Part model, mm, in its own coordinate system. A direction names the side the tool comes from. Round coordinates to 2 decimals unless told otherwise and drop trailing zeros. Order: outer loops, then holes, each group sorted by start corner. A loop starts at its lowest first (then second) coordinate and runs counter-clockwise, first axis right, second up. Notation, with made-up numbers: (2, 2.5) - (42, 2.5) arc R13 ccw to (42, 23.5) - close; hole circle Ø5 at (86, -39.75). An arc over 180 degrees is marked (long way). Answer as a JSON object with one key per item and string values.
```python
from build123d import *

# Parameters (mm, degrees)
FILLET1_R      = 0.1
FILLET2_R      = 0.12
CHAMFER1_SIZE  = 0.2
EXTRUDE1_DEPTH = 1.1


with BuildPart() as part:
    # Sketch1 → Revolve1 (revolve)
    with BuildSketch(Plane.XY, mode=Mode.PRIVATE) as revolve1_sk:
        Polygon((2.5, 1.25), (2.5, 0), (4.279914881, 0), (27.5, 0), (27.5, 1.25), align=None)
        Polygon((0, 2.25), (0, 0), (2.5, 0), (2.5, 1.25), (2.5, 2.25), align=None)
    revolve(revolve1_sk.sketch.rotate(Axis((0, 0, 0), (1, 0, 0)), 90), axis=Axis((0, 0, 0), (1, 0, 0)))

    # Fillet1
    fillet1_edges = [part.edges().sort_by_distance(p)[0] for p in [
        (2.5, 0, -1.25),
    ]]
    fillet(fillet1_edges, radius=FILLET1_R)

    # Fillet2
    fillet2_edges = [part.edges().sort_by_distance(p)[0] for p in [
        (0, 0, -2.25),
    ]]
    fillet(fillet2_edges, radius=FILLET2_R)

    # Chamfer1
    chamfer1_edges = [part.edges().sort_by_distance(p)[0] for p in [
        (27.5, 0, -1.25),
    ]]
    chamfer(chamfer1_edges, length=CHAMFER1_SIZE)

    # Sketch2 → Extrude1 (cut)
    with BuildSketch(Plane.ZY):
        Polygon((0, 1.154700538), (-1, 0.577350269), (-1, -0.577350269), (0, -1.154700538), (1, -0.577350269), (1, 0.577350269), align=None)
    extrude(amount=-EXTRUDE1_DEPTH, mode=Mode.SUBTRACT)


solid = part.part
```
Item 1: Tool access for faces 1 (the flat face through (27.5, 0, 0)), 2 (the flat face through (0.5, 0, -1)), 3 (the cylindrical face through (14.78, -0.05, -1.25)): list every direction of +Z, -Z, +X, -X, +Y, -Y with a clear straight run to the whole face (end or side of a thin tool).
Taken from the geometry:
{"face 1": "+Z, -Z, +X, +Y, -Y", "face 2": "-X", "face 3": "+X"}
Item 2: Cut at A-A (y = 0). Write the cut outline in (x, z), plus the area to 3 significant figures.
Taken from the geometry:
{"outline": "(0, -2.13) arc R0.12 ccw to (0.12, -2.25) - (2.5, -2.25) - (2.5, -1.35) arc R0.1 cw to (2.6, -1.25) - (27.3, -1.25) - (27.5, -1.05) - (27.5, 1.05) - (27.3, 1.25) - (2.6, 1.25) arc R0.1 cw to (2.5, 1.35) - (2.5, 2.25) - (0.12, 2.25) arc R0.12 ccw to (0, 2.13) - (0, 1) - (1.1, 1) - (1.1, -1) - (0, -1) - close", "area": "71.5 mm2"}
Item 3: Cut at B-B (x = 11.25). Write the cut outline in (y, z), plus the area to 3 significant figures.
Taken from the geometry:
{"outline": "circle Ø2.5 at (0, 0)", "area": "4.91 mm2"}
Item 4: Probe L1, parallel to X at y = 0.45, z = 1.3; L2, parallel to X at y = 0.1, z = -0.6; L3, parallel to Z at x = 2, y = -1.4. List the from-to ranges inside material, lowest first. Write a range as from..to.
Taken from the geometry:
{"L1": "0..2.5", "L2": "1.1..27.5", "L3": "-1.76..1.76"}
Item 5: Two-plate mould, pull along Z, no slides. Class faces 4 (the cylindrical face through (1.29, -1.52, -1.66)), 5 (the flat face through (2.5, 1.5, -0.5)), 6 (the flat face through (0.54, 0.87, -0.49)): pulls with the +Z half, pulls with the -Z half, needs draft (parallel to the pull), parting line crosses it, or undercut.
Taken from the geometry:
{"face 4": "parting line crosses it", "face 5": "needs draft", "face 6": "undercut"}
